The listing builds one solid part. Answer for the finished solid, in the listing's coordinates (mm). A direction names the side the tool comes from. Coordinates: 2 decimals unless noted, no trailing zeros. Order: outer loops, then holes, each group sorted by start corner. A loop starts at its lowest first (then second) coordinate and runs counter-clockwise, first axis right, second up.
```python
from build123d import *

# Parameters (mm, degrees)
BOSS_EXTRUDE1_DEPTH = 5
BOSS_EXTRUDE2_DEPTH = 0.5
FILLET1_R           = 0.5
FILLET2_R           = 0.25
SKETCH3_R           = 1.75
CUT_EXTRUDE1_DEPTH  = 0.75


with BuildPart() as part:
    # Sketch1 → Boss-Extrude1 (new body)
    with BuildSketch(Plane.XY):
        Polygon((0, 5.629165125), (-4.875, -2.814582562), (4.875, -2.814582562), align=None)
    extrude(amount=BOSS_EXTRUDE1_DEPTH)

    # Sketch2 → Boss-Extrude2 (add)
    with BuildSketch(Plane(origin=(0, 0, 0), x_dir=(-1, 0, 0), z_dir=(0, 0, -1))):
        Polygon((0, 8.082903769), (-7, -4.041451884), (7, -4.041451884), align=None)
    extrude(amount=BOSS_EXTRUDE2_DEPTH)

    # Fillet1
    fillet1_edges = [part.edges().sort_by_distance(p)[0] for p in [
        (-7, -4.041451884, -0.25),
        (0, 8.082903769, -0.25),
        (7, -4.041451884, -0.25),
    ]]
    fillet(fillet1_edges, radius=FILLET1_R)

    # Fillet2
    fillet2_edges = [part.edges().sort_by_distance(p)[0] for p in [
        (4.875, -2.814582562, 2.5),
        (-4.875, -2.814582562, 2.5),
        (0, 5.629165125, 2.5),
    ]]
    fillet(fillet2_edges, radius=FILLET2_R)

    # Sketch3 → Cut-Extrude1 (cut)
    with BuildSketch(Plane(origin=(0, 0, -0.5), x_dir=(-1, 0, 0), z_dir=(0, 0, -1))):
        Circle(SKETCH3_R)
    extrude(amount=-CUT_EXTRUDE1_DEPTH, mode=Mode.SUBTRACT)


solid = part.part
```
(1) Find section D-D (y = 1). Write down the section's boundary in (x, z), and give its area (3 significant figures).
(2) Find section B-B (x = 0). Write down the section's boundary in (y, z).
(3) Find section C-C (y = 4.25). Write down the section's boundary in (x, z).
(4) Find section A-A (z = 3.65). Write down the section's boundary in (x, y).
(5) For faces 4 (the face through (3.457, 2.095, -0.246)), 5 (the face through (0, 2, -0.5)), 6 (the face through (2.47, 1.35, 2.46)), 7 (the face through (0, -2.815, 2)), 8 (the face through (0, 0, 0.25)), determine the directions among +Z, -Z, +X, -X, +Y, -Y from which every point of the face is accessible in a straight line to the end or side of a thin tool.
(6) The mould has two halves that part along Y. Classify faces 1 (the face through (-2.406, 1.461, 2.465)), 2 (the face through (0, -3, 0)), 3 (the face through (-1.617, -0.67, -0.13)): released by +Y, released by -Y, zero draft, split by the parting line, or undercut.
(7) Consider line 1 (Z direction, x = 5.5, y = -2.5); line 2 (X direction, y = 0.25, z = 0.15); line 3 (X direction, y = -0.5, z = 0.2). Determine where each line is inside the solid, lowest interval first.
(8) Each of these flat-tipped pins is pushed along its axis until it touches: pin 1 Ø1.5 at (x, z) = (0.5, 3.5) entering from -Y; pin 2 Ø1.5 at (y, z) = (2.5, 1) entering from -X; pin 3 Ø1.5 at (y, z) = (1, 2) entering from +X. Where does it stop, or does it pass through?
Findings below:
1. outline: (-4.09, -0.5) - (-1.44, -0.5) - (-1.44, 0.25) - (1.44, 0.25) - (1.44, -0.5) - (4.09, -0.5) - (4.09, 0) - (2.67, 0) - (2.67, 5) - (-2.67, 5) - (-2.67, 0) - (-4.09, 0) - close
1. area: 28.7 mm2
2. outline: (-4.04, -0.5) - (-1.75, -0.5) - (-1.75, 0.25) - (1.75, 0.25) - (1.75, -0.5) - (7.58, -0.5) - (7.58, 0) - (5.38, 0) - (5.38, 5) - (-2.81, 5) - (-2.81, 0) - (-4.04, 0) - close
3. outline: (-2.21, -0.5) - (2.21, -0.5) - (2.21, 0) - (0.8, 0) - (0.8, 5) - (-0.8, 5) - (-0.8, 0) - (-2.21, 0) - close
4. outline: (-4.66, -2.44) arc R0.25 ccw to (-4.44, -2.81) - (4.44, -2.81) arc R0.25 ccw to (4.66, -2.44) - (0.22, 5.25) arc R0.25 ccw to (-0.22, 5.25) - close
5. face 4: +Z, -Z, +X, +Y
5. face 5: -Z, +X, -X, +Y, -Y
5. face 6: +Z, +X, +Y
5. face 7: +Z, +X, -X, -Y
5. face 8: -Z
6. face 1: released by +Y
6. face 2: zero draft
6. face 3: undercut
7. line 1: z = -0.5 to 0
7. line 2: x = -3.11 to -1.73, 1.73 to 3.11
7. line 3: x = -3.54 to -1.68, 1.68 to 3.54
8. pin 1: stops at y = -2.81
8. pin 2: stops at x = -2.24
8. pin 3: stops at x = 3.11
